Can you work these out from the model? Positions are in its coordinate system, mm. Face numbers are marked on the shaded views. A direction names the side the tool comes from. Coordinates: 2 decimals unless noted, no trailing zeros. Write each loop counter-clockwise with the first axis right and the second up, starting at its lowest first coordinate (ties: lowest second). Pieces come first, ordered by that corner, then holes. Notation, with made-up numbers: (-29.75, 3) - (20.25, 3) arc R21 cw to (20.25, 20) - close; hole circle Ø9 at (78, -11). An arc over 180 degrees is marked (long way). Write each question's results on one line, items separated by ' | '. Start each with the question number.
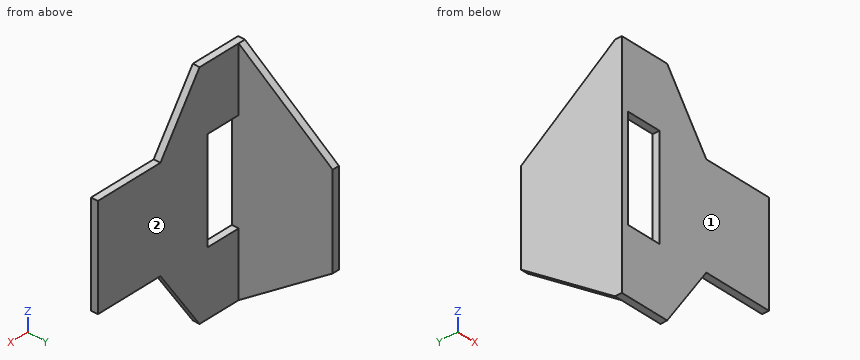
```python
from build123d import *

# Parameters (mm, degrees)
BOSS_EXTRUDE1_DEPTH = 4
BOSS_EXTRUDE3_DEPTH = 4


with BuildPart() as part:
    # Sketch1 → Boss-Extrude1 (new body)
    with BuildSketch(Plane(origin=(0, 0, 0), x_dir=(1, 0, 0), z_dir=(0, 1, 0))):
        Polygon((-15, 30), (25, 30), (25, -30), (-15, -30), (-40, -68), (-65, -68), (-65, -30), (-45, -30), (-45, 30), (-65, 30), (-65, 68), (-40, 68), align=None)
    extrude(amount=BOSS_EXTRUDE1_DEPTH)

    # Sketch3 → Boss-Extrude3 (add)
    with BuildSketch(Plane.ZY.offset(65)):
        Polygon((-68, 0), (-68, 4), (-27.5, 60), (27.5, 60), (68, 4), (68, 0), align=None)
    extrude(amount=BOSS_EXTRUDE3_DEPTH)


solid = part.part
```
Q1. If we section it at D-D (y = 28): Please give me the cut outline in (x, z).
Q2. If we section it at B-B (x = -61): Please give me the cut outline in (y, z), then the cut area to 3 significant figures.
Q3. If we section it at C-C (x = -23): Please give me the cut outline in (y, z), then the cut area to 3 significant figures.
Q4. If we section it at A-A (z = 0.5): Please give me the cut outline in (x, y).
Q5. I need wall thicknesses on line 1 along Y through (x, z) = (-39, -33); line 2 along X through (y, z) = (25.5, 40). Which ranges of each line are inside material? Lowest first, please. Write a range as from..to.
Q6. I'm going to push flat-ended pins straight in: pin 1 Ø4.5 at (x, y) = (4, 1) entering from -Z; pin 2 Ø1.2 at (x, y) = (-3.5, 1.5) entering from +Z; pin 3 Ø8 at (x, z) = (-36, -35) entering from +Y. Where does each tip first touch, or does it pass through?
Q7. For the marked faces 1 and 2, which set-ups out of +Z, -Z, +X, -X, +Y, -Y let a thin tool reach every point of the face, with its end or its side?
Answer list:
1) outline: (-69, -50.64) - (-65, -50.64) - (-65, 50.64) - (-69, 50.64) - close
2) outline: (0, -68) - (4, -68) - (4, -30) - (0, -30) - close; (0, 30) - (4, 30) - (4, 68) - (0, 68) - close | area: 304 mm2
3) outline: (0, -42.16) - (4, -42.16) - (4, 42.16) - (0, 42.16) - close | area: 337 mm2
4) outline: (-69, 0) - (-65, 0) - (-65, 60) - (-69, 60) - close; (-45, 0) - (25, 0) - (25, 4) - (-45, 4) - close
5) line 1: y = 0..4 | line 2: x = -69..-65
6) pin 1: stops at z = -30 | pin 2: stops at z = 30 | pin 3: stops at y = 4
7) face 1: +Z, -Z, +X, -X, -Y | face 2: +Z, -Z, +X, +Y
